```python
from build123d import *

# Parameters (mm, degrees)
BOSS_EXTRUDE1_DEPTH = 35
BOSS_EXTRUDE2_REACH = 94.65
SKETCH5_W           = 3
SKETCH5_H           = 10
BOSS_EXTRUDE3_REACH = 54.382
SKETCH6_W           = 3
SKETCH6_H           = 10.000117819
SKETCH7_W           = 3
SKETCH7_H           = 10
BOSS_EXTRUDE4_DEPTH = 52.35


with BuildPart() as part:
    # Sketch1 → Boss-Extrude1 (new body)
    with BuildSketch(Plane.XY):
        Polygon((-75.5, 3.5), (75.5, 3.5), (75.5, -3.5), (23.15, -3.5), (23.15, -13.5), (17.15, -13.5), (17.15, -3.5), (-17.15, -3.5), (-17.2, -13.5), (-23.199999999, -13.499882182), (-23.151457837, -3.5), (-75.5, -3.5), align=None)
    extrude(amount=BOSS_EXTRUDE1_DEPTH)

    # Boss-Extrude2: up to this face of the body (flat: up to its plane)
    boss_extrude2_end = Plane(part.part.faces().sort_by_distance((-17.175, -8.5, 17.5))[0])
    # Sketch5 → Boss-Extrude2 (add, up to the picked face)
    with BuildSketch(Plane.ZY.offset(-17.15), mode=Mode.PRIVATE) as boss_extrude2_sk1:
        with Locations((33.5, -8.5)):
            Rectangle(SKETCH5_W, SKETCH5_H)
    boss_extrude2_tool1 = split(extrude(boss_extrude2_sk1.sketch, amount=BOSS_EXTRUDE2_REACH, mode=Mode.PRIVATE), bisect_by=boss_extrude2_end, keep=Keep.BOTH, mode=Mode.PRIVATE)
    add(boss_extrude2_tool1.solids().sort_by_distance((17.15, -8.5, 33.5))[0])

    # Boss-Extrude3: up to this face of the body (flat: up to its plane)
    boss_extrude3_end = Plane(part.part.faces().sort_by_distance((-75.5, 0, 17.5))[0])
    # Sketch6 → Boss-Extrude3 (add, up to the picked face)
    with BuildSketch(Plane(origin=(-23.133922754, 0.112298384, 0), x_dir=(0, 0, 1), z_dir=(-0.999988218, 0.004854216, 0)), mode=Mode.PRIVATE) as boss_extrude3_sk1:
        with Locations((33.5, -8.612399854)):
            Rectangle(SKETCH6_W, SKETCH6_H)
    boss_extrude3_tool1 = split(extrude(boss_extrude3_sk1.sketch, amount=BOSS_EXTRUDE3_REACH, mode=Mode.PRIVATE), bisect_by=boss_extrude3_end, keep=Keep.BOTH, mode=Mode.PRIVATE)
    add(boss_extrude3_tool1.solids().sort_by_distance((-23.175729, -8.5, 33.5))[0])

    # Sketch7 → Boss-Extrude4 (add)
    with BuildSketch(Plane(origin=(23.15, 0, 0), x_dir=(0, 0, -1), z_dir=(1, 0, 0))):
        with Locations((-33.5, -8.5)):
            Rectangle(SKETCH7_W, SKETCH7_H)
    extrude(amount=BOSS_EXTRUDE4_DEPTH)


solid = part.part
```
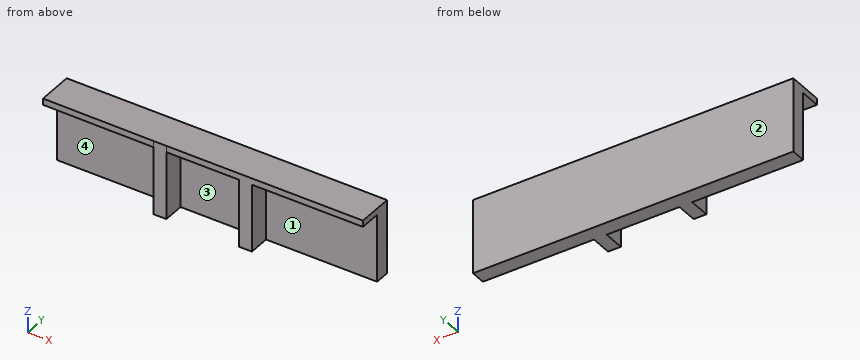
Verification items for the finished model (mm, model axes). Face numbers are marked on the shaded views. A direction names the side the tool comes from. Coordinates: 2 decimals unless noted, no trailing zeros. Write each loop counter-clockwise with the first axis right and the second up, starting at its lowest first coordinate (ties: lowest second). Pieces come first, ordered by that corner, then holes. Notation, with made-up numbers: (24.25, -21) - (67.25, -21) arc R15 ccw to (67.25, -12) - close; hole circle Ø5 at (-21.5, -19.5). An arc over 180 degrees is marked (long way). Write item = value, one per line.
Q1. Cross-section at B-B (y = -9.25). Enter the section's corners in (x, z).
Answer:
outline = (-75.5, 32) - (-23.18, 32) - (-23.18, 0) - (-17.18, 0) - (-17.18, 32) - (17.15, 32) - (17.15, 0) - (23.15, 0) - (23.15, 32) - (75.5, 32) - (75.5, 35) - (-75.5, 35) - close
Q2. Mould release check, pull along X, two halves, no side actions. Record for the marked faces 3 and 4: released by +X, released by -X, zero draft, split by the parting line, or undercut.
Answer:
face_3 = undercut
face_4 = zero draft
Q3. Cross-section at C-C (x = 10). Enter the section's corners in (y, z), plus the area to 3 significant figures.
Answer:
outline = (-13.5, 32) - (-3.5, 32) - (-3.5, 0) - (3.5, 0) - (3.5, 35) - (-13.5, 35) - close
area = 275 mm²
Q4. Cross-section at A-A (z = 20.5). Enter the section's corners in (x, y), plus the area to 3 significant figures.
Answer:
outline = (-75.5, -3.5) - (-23.15, -3.5) - (-23.2, -13.5) - (-17.2, -13.5) - (-17.15, -3.5) - (17.15, -3.5) - (17.15, -13.5) - (23.15, -13.5) - (23.15, -3.5) - (75.5, -3.5) - (75.5, 3.5) - (-75.5, 3.5) - close
area = 1,180 mm²
Q5. Material ranges on L1, parallel to X at y = -4, z = 18; L2, parallel to Y at x = 40.5, z = 3; L3, parallel to Z at x = -32.5, y = -5.75, recorded low to high. Write a range as from..to.
Answer:
L1 = -23.15..-17.15, 17.15..23.15
L2 = -3.5..3.5
L3 = 32..35
Q6. Cross-section at D-D (x = -52). Enter the section's corners in (y, z).
Answer:
outline = (-13.36, 32) - (-3.5, 32) - (-3.5, 0) - (3.5, 0) - (3.5, 35) - (-13.36, 35) - close
Q7. Go/stop test with flat-tipped pins: pin 1 Ø1.5 at (x, y) = (-5, -11) entering from -Z; pin 2 Ø5 at (y, z) = (-9, 20) entering from -X; pin 3 Ø9.5 at (x, z) = (-39.5, 17) entering from -Y. Record where each tip stops, or that it passes through.
Answer:
pin_1 = 32
pin_2 = -23.19
pin_3 = -3.5
Q8. Access from +Z, -Z, +X, -X, +Y, -Y to the whole of each face (thin tool, end or side, straight path). Record for the marked faces 1 and 2.
Answer:
face_1 = -Z, +X, -Y
face_2 = +Z, -Z, +X, -X, +Y
